Autodesk Inventor part; units mm, degrees
ref_plane "YZ Plane" through (0, 0, 0) normal (1, 0, 0) x (0, 1, 0)
ref_plane "XZ Plane" through (0, 0, 0) normal (0, 1, 0) x (-1, 0, 0)
ref_plane "XY Plane" through (0, 0, 0) normal (0, 0, 1) x (1, 0, 0)
sketch "Sketch3" plane through (0, 0, 0) normal (1, 0, 0) x (0, 1, 0)
  line L0 (0, -27.432) -> (0, -56.388)
  line L1 (0, -56.388) -> (50.8, -19.4796)
  line L2 (50.8, -19.4796) -> (50.8, 9.4764)
  line L3 (7.4884, -44.196) -> (-9.6833, -44.196) construction
  line L4 (0, -27.432) -> (50.8, 9.4764)
  line L5 (0, 56.388) -> (50.8, 19.4796)
  line L6 (50.8, 19.4796) -> (50.8, -10.7464)
  line L7 (0, 56.388) -> (0, 26.162)
  line L8 (0, 26.162) -> (50.8, -10.7464)
  point P0 (0, 0)
  dimension "d23" = 54
  dimension "d25" = 44.196
  dimension "d26" = 16.764
  dimension "d27" = 12.192
  dimension "d28" = 50.8
  dimension "d33" = 0
  dimension "d34" = 54
  dimension "d35" = 50.8
  dimension "d36" = 53.594
  dimension "d37" = 112.776
extrude "Extrusion1" add sketch "Sketch3" along normal blind 38.1
sketch "Sketch5" plane through (0, 50.8, 19.4796) normal (0, 1, 0) x (1, 0, 0)
  circle A0 centre (19.05, 19.4775) radius 20.701
  line L0 (0, 38.9593) -> (38.1, 38.9593)
  line L1 (38.1, 38.9593) -> (38.1, 0)
  line L2 (0, 0) -> (38.1, 0)
  line L3 (38.1, 0) -> (0, 0)
  line L4 (0, 0) -> (0, 38.9593)
  line L5 (0, 38.9593) -> (38.1, 38.9593)
  line L6 (38.1, 38.9593) -> (38.1, 0)
  point P0 (0, 19.4796)
  dimension "d40" = 41.402
  dimension "d42" = 19.05
  dimension "d43" = 38.9593
  dimension "d44" = 19.4818
extrude "Extrusion2" add sketch "Sketch5" along normal blind 22.098 contours A0 L1 | L1 A0 L2 L4 L0 | L0 A0 | A0 L2 | L4 A0
extrude "Extrusion3" add sketch "Sketch5" against normal blind 28.448 contours A0 L1 | L1 A0 L2 L4 L0 | L0 A0 | A0 L2 | L4 A0
sketch "Sketch8" plane through (19.05, 72.898, 0.0022) normal (0, 1, 0) x (1, 0, 0)
  circle A0 centre (0, 0) radius 17.526
  circle A1 centre (0, 0) radius 20.701
  point P0 (-19.05, 0.0022)
  dimension "d50" = 35.052
extrude "Extrusion4" add sketch "Sketch8" along normal blind 2.54 contours A0
sketch "Sketch9" plane through (19.05, 75.438, 0.0022) normal (0, 1, 0) x (1, 0, 0)
  circle A0 centre (0, 0) radius 19.05
  circle A1 centre (0, 0) radius 17.526
  point P0 (-19.05, 0.0022)
  dimension "d53" = 38.1
extrude "Extrusion5" add sketch "Sketch9" along normal blind 2.286 contours A0 | A1
sketch "Sketch10" plane through (19.05, 77.724, 0.0022) normal (0, 1, 0) x (1, 0, 0)
  circle A0 centre (0, 0) radius 5.08
  circle A1 centre (0, 0) radius 19.05
  point P0 (-19.05, 0.0022)
  dimension "d56" = 10.16
extrude "Extrusion6" add sketch "Sketch10" along normal blind 40.64 contours A0
properties part number "gear mount"
Geometry check sheet. Reference: the model listing, model coordinates, mm. A direction names the side the tool comes from. Give positions to 0.01 mm unless a question says otherwise; leave off trailing zeros. Loops run counter-clockwise (first coordinate to the right, second up) from the corner with the lowest first, then second, coordinate; pieces in that order, holes last. Notation, with made-up numbers: M -17.75,88 L 36.25,88 A22 cw 36.25,104 Z; hole C 74,-37.75 d9. An arc over 180 degrees is marked long. Write item = value, one per line. Start each with the question number.
1. Section check A-A, the plane y = 15. Enter the section's corners in (x, z).
2. Section check C-C, the plane y = 35.5. Enter the section's corners in (x, z).
3. Draft check along Z on faces 6 (the face through (18.78, 12.25, 17.26)), 7 (the face through (19, 22.352, -1)), 8 (the face through (0, 19, 27)), 9 (the face through (18.783, 25.044, 38.192)). Enter one of: +Z half, -Z half, draft (parallel to the pull), parting line (faces both ways), or undercut.
4. Section check B-B, the plane x = 5. Enter the section's corners in (y, z).
5. Thickness scan on probe 1 along Y at (x, z) = (21, 4.5); probe 2 along X at (y, z) = (31, -22); probe 3 along Z at (x, y) = (7.5, 6). Record the ranges inside material, lowest first.
6. Tool access check on faces 1 (the face through (2, 72.898, -5)), 2 (the face through (38.1, 25, -27)), 3 (the face through (3, 50.8, 16)), 4 (the face through (38.1, 19, 27)), 5 (the face through (35, 50.8, 16)). Record the directions out of +Z, -Z, +X, -X, +Y, -Y that give a thin tool (end or side, any length) a straight path to the whole face; none if there is none.
7. Section check D-D, the plane z = 42.5. Enter the section's corners in (x, y), plus the area to 3 significant figures.
8. Go/stop test with flat-tipped pins: P1, Ø10, axis at x = 23, z = 32, coming from the +Y side; P2, Ø8, axis at x = 7.5, y = 84, coming from the +Z side; P3, Ø5.5, axis at x = 30.5, z = -12, coming from the +Y side; P4, Ø3, axis at x = 34, y = 15, coming from the +Z side. Record where each tip stops, or that it passes through.
Values follow:
q1.outline = M 0,-45.49 L 38.1,-45.49 L 38.1,-16.53 L 0,-16.53 Z; M 0,15.26 L 38.1,15.26 L 38.1,45.49 L 0,45.49 Z
q2.outline = M 0,-30.6 L 38.1,-30.6 L 38.1,-8.1 A20.7 ccw 38.1,8.1 L 38.1,30.6 L 0,30.6 L 0,8.1 A20.7 ccw 0,-8.1 Z
q3.face_6 = undercut
q3.face_7 = undercut
q3.face_8 = draft
q3.face_9 = +Z half
q4.outline = M 0,-56.39 L 50.8,-19.48 L 50.8,-15.2 L 72.9,-15.2 L 72.9,-10.47 L 75.44,-10.47 L 75.44,-12.86 L 77.72,-12.86 L 77.72,12.87 L 75.44,12.87 L 75.44,10.48 L 72.9,10.48 L 72.9,15.21 L 50.8,15.21 L 50.8,19.48 L 0,56.39 L 0,26.16 L 22.35,9.92 L 22.35,-11.19 L 0,-27.43 Z
q5.probe_1 = 22.35 to 118.36
q5.probe_2 = 0 to 38.1
q5.probe_3 = -52.03 to -23.07, 21.8 to 52.03
q6.face_1 = none
q6.face_2 = -Z, +X, +Y, -Y
q6.face_3 = +Z, -X, +Y
q6.face_4 = +Z, +X, +Y, -Y
q6.face_5 = +Z, +X, +Y
q7.outline = M 0,0 L 38.1,0 L 38.1,19.12 L 0,19.12 Z
q7.area = 728 mm^2
q8.P1 = 40.45
q8.P2 = through
q8.P3 = 77.72
q8.P4 = 46.58
